Build history of the part. All positions in model axes, mm. Round coordinates to 2 decimals unless told otherwise and drop trailing zeros. Order: outer loops, then holes, each group sorted by start corner. A loop starts at its lowest first (then second) coordinate and runs counter-clockwise, first axis right, second up. Notation, with made-up numbers: (83.5, 62.5) -> (103.5, 62.5) arc R31 cw to (103.5, 87.5) -> close; hole circle Ø1 at (-38.5, 60.5). An arc over 180 degrees is marked (long way). Write item = value, one per line.
from build123d import *

# Parameters (mm, degrees)
BOSS_EXTRUDE1_DEPTH = 5


with BuildPart() as part:
    # Sketch1 → Boss-Extrude1 (new body)
    with BuildSketch(Plane.XY):
        with BuildLine():
            Line((38, -50), (75, -50))
            Line((75, -50), (75, 90))
            Line((75, 90), (-75, 90))
            Line((-75, 90), (-75, -50))
            Line((-75, -50), (32, -50))
            ThreePointArc((32, -50), (35, -47), (38, -50))
        make_face()
        with BuildLine():
            Line((-75, -90), (75, -90))
            Line((75, -90), (75, -50))
            Line((75, -50), (38, -50))
            ThreePointArc((38, -50), (35, -53), (32, -50))
            Line((32, -50), (-75, -50))
            Line((-75, -50), (-75, -90))
        make_face()
    extrude(amount=BOSS_EXTRUDE1_DEPTH)


solid = part.part
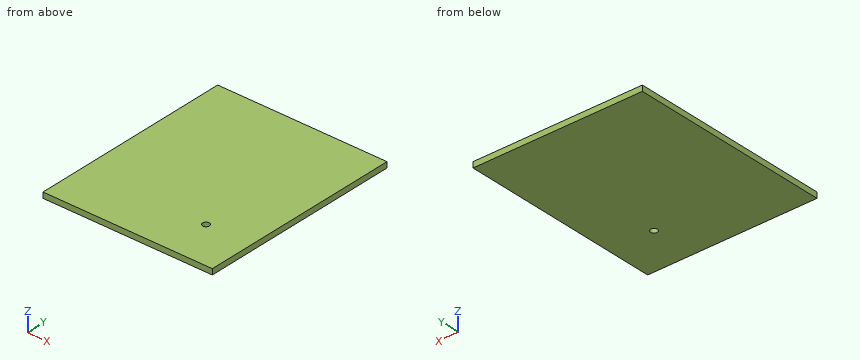
Q1. Probe probe 1 along X at (y, z) = (-50, 1.4); probe 2 along Y at (x, z) = (34.5, 1.85). List the from-to ranges inside material, lowest first.
Check values:
probe_1 = -75 to 32, 38 to 75
probe_2 = -90 to -52.96, -47.04 to 90
Q2. Cut at B-B, the plane y = -50. List the corners of the cut face in (x, z), and give its area (3 significant figures).
Check values:
outline = (-75, 0) -> (32, 0) -> (32, 5) -> (-75, 5) -> close; (38, 0) -> (75, 0) -> (75, 5) -> (38, 5) -> close
area = 720 mm²
Q3. Cut at A-A, the plane x = 35. List the corners of the cut face in (y, z), and give its area (3 significant figures).
Check values:
outline = (-90, 0) -> (-53, 0) -> (-53, 5) -> (-90, 5) -> close; (-47, 0) -> (90, 0) -> (90, 5) -> (-47, 5) -> close
area = 870 mm²
